The listing builds one solid part. Answer for the finished solid, in the listing's coordinates (mm). Face numbers are marked on the shaded views. A direction names the side the tool comes from. Give positions to 0.01 mm unless a question says otherwise; leave off trailing zeros. Loops run counter-clockwise (first coordinate to the right, second up) from the corner with the lowest first, then second, coordinate; pieces in that order, holes last. Notation, with made-up numbers: (-17.5, -13) - (-8.5, -13) arc R31 ccw to (-8.5, 17) - close; hole circle Ø8 at (15.5, 41). An arc over 180 degrees is marked (long way). One line per item, written item: value. Start each with the question number.
from build123d import *

# Parameters (mm, degrees)
SKETCH_1_R      = 1.55
SKETCH_1_R_2    = 0.7
EXTRUDE_1_DEPTH = 3
FILLET_1_R      = 1


with BuildPart() as part:
    # 草图1 → 凸台-拉伸1 (new body)
    with BuildSketch(Plane.XY):
        Polygon((-5, 10), (5, 10), (5, 0), (10, 0), (10, -10), (5, -10), (-5, -10), (-10, -10), (-10, 0), (-5, 0), align=None)
        with Locations((-6.45, -5)):
            Circle(SKETCH_1_R, mode=Mode.SUBTRACT)
        with Locations((6.45, -5)):
            Circle(SKETCH_1_R, mode=Mode.SUBTRACT)
        Circle(SKETCH_1_R_2, mode=Mode.SUBTRACT)
        with Locations((0, 7)):
            Circle(SKETCH_1_R_2, mode=Mode.SUBTRACT)
    extrude(amount=EXTRUDE_1_DEPTH)

    # 圆角1
    fillet_1_edges = [part.edges().sort_by_distance(p)[0] for p in [
        (-10, -10, 1.5),
        (-10, 0, 1.5),
        (-5, 0, 1.5),
        (-5, 10, 1.5),
        (5, 10, 1.5),
        (5, 0, 1.5),
        (10, 0, 1.5),
        (10, -10, 1.5),
    ]]
    fillet(fillet_1_edges, radius=FILLET_1_R)


solid = part.part
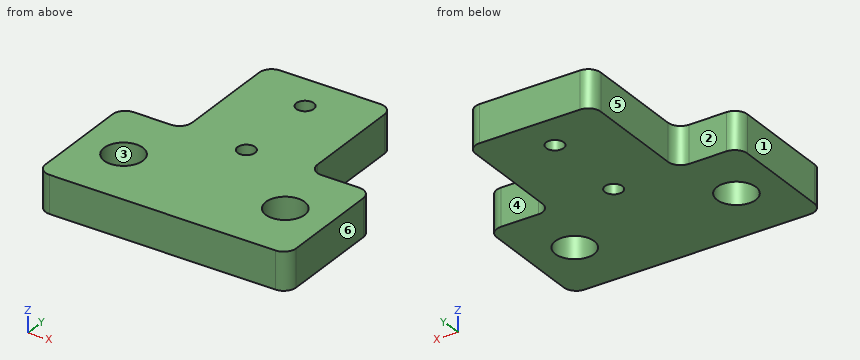
1. A cutting plane is placed at D-D (y = -5). Determine the outline of the cut face in (x, z), plus the area to 3 significant figures.
2. Find the intervals of material crossed by L1, parallel to X at y = -5.75, z = 0.3; L2, parallel to Y at x = 6.45, z = 2.2; L3, parallel to Y at x = 7, z = 2.55, in increasing order. Write a range as [from, to].
3. Determine the mould class of the marked faces 1, 2 and 3 for opening direction Y: released by +Y, released by -Y, zero draft, split by the parting line, or undercut.
4. Flat-ended cylindrical pins translate along their axes: pin 1 (1.5 mm diameter, centred on x = 7, z = 1.5, fed in from +Y); pin 2 (0.9 mm diameter, centred on y = 3.5, z = 1, fed in from -X). Find the tip coordinate at first contact, or state that the pin passes through.
5. A cutting plane is placed at C-C (x = -6.45). Determine the outline of the cut face in (y, z), plus the area to 3 significant figures.
6. For the marked faces 4, 5 and 6, determine the directions among +Z, -Z, +X, -X, +Y, -Y from which every point of the face is accessible in a straight line to the end or side of a thin tool.
7. A cutting plane is placed at A-A (y = 7). Determine the outline of the cut face in (x, z).
8. A cutting plane is placed at B-B (z = 0.5). Determine the outline of the cut face in (x, y), plus the area to 3 significant figures.
Results below:
1. outline: (-10, 0) - (-8, 0) - (-8, 3) - (-10, 3) - close; (-4.9, 0) - (4.9, 0) - (4.9, 3) - (-4.9, 3) - close; (8, 0) - (10, 0) - (10, 3) - (8, 3) - close
1. area: 41.4 mm^2
2. L1: x = [-10, -7.81], [-5.09, 5.09], [7.81, 10]
2. L2: y = [-10, -6.55], [-3.45, 0]
2. L3: y = [-10, -6.45], [-3.55, 0]
3. face 1: zero draft
3. face 2: released by +Y
3. face 3: undercut
4. pin 1: stops at y = 0
4. pin 2: stops at x = -5
5. outline: (-10, 0) - (-6.55, 0) - (-6.55, 3) - (-10, 3) - close; (-3.45, 0) - (0, 0) - (0, 3) - (-3.45, 3) - close
5. area: 20.7 mm^2
6. face 4: +Z, -Z, +X, +Y
6. face 5: +Z, -Z, -X, +Y
6. face 6: +Z, -Z, +X, +Y, -Y
7. outline: (-5, 0) - (-0.7, 0) - (-0.7, 3) - (-5, 3) - close; (0.7, 0) - (5, 0) - (5, 3) - (0.7, 3) - close
8. outline: (-10, -9) arc R1 ccw to (-9, -10) - (9, -10) arc R1 ccw to (10, -9) - (10, -1) arc R1 ccw to (9, 0) - (6, 0) arc R1 cw to (5, 1) - (5, 9) arc R1 ccw to (4, 10) - (-4, 10) arc R1 ccw to (-5, 9) - (-5, 1) arc R1 cw to (-6, 0) - (-9, 0) arc R1 ccw to (-10, -1) - close; hole circle Ø3.1 at (-6.45, -5); hole circle Ø1.4 at (0, 0); hole circle Ø1.4 at (0, 7); hole circle Ø3.1 at (6.45, -5)
8. area: 281 mm^2
